```python
from build123d import *

# Parameters (mm, degrees)
BOSS_EXTRUDE1_DEPTH = 21.15
BOSS_EXTRUDE1_TAPER = 1
SKETCH2_R           = 18.1
BOSS_EXTRUDE2_DEPTH = 12.75
SKETCH3_R           = 1.25
CUT_EXTRUDE1_DEPTH  = 35.529733564
FILLET1_R           = 1
CUT_EXTRUDE2_DEPTH  = 1
CIRPATTERN1_COUNT   = 8


with BuildPart() as part:
    # Sketch1 → Boss-Extrude1 (new body)
    with BuildSketch(Plane.XY):
        with BuildLine():
            ThreePointArc((-14.3, 19.3), (-17.835533906, 17.835533906), (-19.3, 14.3))
            Line((-19.3, 14.3), (-19.3, -14.3))
            ThreePointArc((-19.3, -14.3), (-17.835533906, -17.835533906), (-14.3, -19.3))
            Line((-14.3, -19.3), (14.3, -19.3))
            ThreePointArc((14.3, -19.3), (17.835533906, -17.835533906), (19.3, -14.3))
            Line((19.3, -14.3), (19.3, 14.3))
            ThreePointArc((19.3, 14.3), (17.835533906, 17.835533906), (14.3, 19.3))
            Line((14.3, 19.3), (-14.3, 19.3))
        make_face()
    extrude(amount=BOSS_EXTRUDE1_DEPTH, taper=BOSS_EXTRUDE1_TAPER)

    # Sketch2 → Boss-Extrude2 (add)
    with BuildSketch(Plane.XY.offset(21.15)):
        Circle(SKETCH2_R)
    extrude(amount=BOSS_EXTRUDE2_DEPTH)

    # Sketch3 → Cut-Extrude1 (cut, through all)
    with BuildSketch(Plane.XY.offset(21.15)):
        with Locations((-15.7, 15.7)):
            Circle(SKETCH3_R)
        with Locations(Location((15.7, 15.7, 0), (0, 0, 180))):
            Circle(SKETCH3_R)
        with Locations((15.7, -15.7)):
            Circle(SKETCH3_R)
        with Locations(Location((-15.7, -15.7, 0), (0, 0, 180))):
            Circle(SKETCH3_R)
    extrude(amount=-CUT_EXTRUDE1_DEPTH, mode=Mode.SUBTRACT)

    # Fillet1
    fillet1_edges = [part.edges().sort_by_distance(p)[0] for p in [
        (17.574488026, -17.574488026, 21.15),
        (18.930825377, 0, 21.15),
        (17.574488026, 17.574488026, 21.15),
        (0, 18.930825377, 21.15),
        (-17.574488026, 17.574488026, 21.15),
        (-18.1, 0, 33.9),
        (-18.930825377, 0, 21.15),
        (-17.574488026, -17.574488026, 21.15),
        (0, -18.930825377, 21.15),
    ]]
    fillet(fillet1_edges, radius=FILLET1_R)

    # Sketch4 → Cut-Extrude2 (cut)
    with BuildSketch(Plane.XY.offset(33.9)):
        with BuildLine():
            ThreePointArc((0, 7.385996988), (-2.142431463, -7.068446712), (4.100641433, 6.143101118))
            ThreePointArc((4.100641433, 6.143101118), (6.838415629, 7.989504917), (9.958635041, 9.070636436))
            ThreePointArc((9.958635041, 9.070636436), (4.702829161, 9.862759424), (0, 7.385996988))
        make_face()
    cut_extrude2 = extrude(amount=-CUT_EXTRUDE2_DEPTH, mode=Mode.SUBTRACT)

    # CirPattern1: Cut-Extrude2 ×8 about axis
    cirpattern1_axis = Axis((0, 0, 0), (0, 0, 1))
    for i in range(1, CIRPATTERN1_COUNT):
        add(cut_extrude2.rotate(cirpattern1_axis, i * 360 / CIRPATTERN1_COUNT), mode=Mode.SUBTRACT)


solid = part.part
```
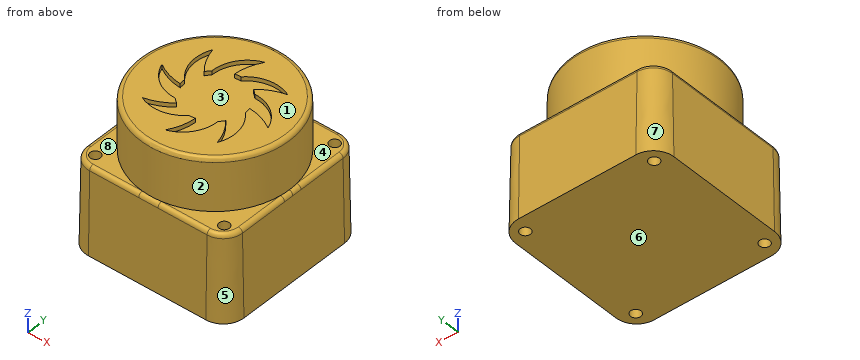
The listing builds one solid part. Answer for the finished solid, in the listing's coordinates (mm). Face numbers are marked on the shaded views. A direction names the side the tool comes from. Coordinates: 2 decimals unless noted, no trailing zeros. Loops run counter-clockwise (first coordinate to the right, second up) from the corner with the lowest first, then second, coordinate; pieces in that order, holes last. Notation, with made-up numbers: (13, -5.75) - (41, -5.75) arc R25 cw to (41, 14.25) - close; hole circle Ø11 at (35.5, 44). An arc over 180 degrees is marked (long way). Use a Markdown table: item, result. Add a question column.
1) The part is cut by section A-A, the plane x = -15.7. State how many separate pieces and enclosed holes the cut face has, and give its area (3 significant figures).
2) The part is cut by section B-B, the plane z = 27. Give the vertices of the cut face in (x, y), and give its area (3 significant figures).
3) Given pin 1 (5 mm diameter, centred on x = -14, z = 22.5, fed in from +Y); pin 2 (1 mm diameter, centred on x = 8.5, z = 8.5, fed in from +Y); pin 3 (1.5 mm diameter, centred on x = -11, z = 12, fed in from +Y); pin 4 (1.5 mm diameter, centred on x = 15.7, y = 15.7, fed in from +Z), each flat-ended and moving along its own axis, determine where each tip first touches the part or whether it passes through.
4) The mould has two halves that part along Y. Classify the marked faces 1, 2 and 3: released by +Y, released by -Y, zero draft, split by the parting line, or undercut.
5) Find the intervals of material crossed by line 1 (X direction, y = -16.5, z = 16.5); line 2 (Y direction, x = -15, z = 8); line 3 (Y direction, x = 15.7, z = 5.5), in increasing order.
6) For the marked faces 4, 5, 6, 7 and 8, determine the directions among +Z, -Z, +X, -X, +Y, -Y from which every point of the face is accessible in a straight line to the end or side of a thin tool.
Here are the results:
| question | item | result |
|---|---|---|
| 1 | separate pieces | 3 |
| 1 | enclosed holes | 0 |
| 1 | area | 922 mm^2 |
| 2 | outline | circle Ø36.2 at (0, 0) |
| 2 | area | 1,030 mm^2 |
| 3 | pin 1 | stops at y = 18.95 |
| 3 | pin 2 | stops at y = 19.16 |
| 3 | pin 3 | stops at y = 19.1 |
| 3 | pin 4 | passes through |
| 4 | face 1 | zero draft |
| 4 | face 2 | split by the parting line |
| 4 | face 3 | undercut |
| 5 | line 1 | x = -18.47 to -16.66, -14.74 to 14.74, 16.66 to 18.47 |
| 5 | line 2 | y = -19.11 to -16.74, -14.66 to 14.66, 16.74 to 19.11 |
| 5 | line 3 | y = -19 to -16.95, -14.45 to 14.45, 16.95 to 19 |
| 6 | face 4 | +Z, +X, +Y |
| 6 | face 5 | +Z, +X, -Y |
| 6 | face 6 | -Z, +X, -X, +Y, -Y |
| 6 | face 7 | +Z, -X, +Y |
| 6 | face 8 | +Z, -X, -Y |
